The model under review builds one solid part; all positions refer to its coordinate system, in mm. A direction names the side the tool comes from. Give positions to 0.01 mm unless a question says otherwise; leave off trailing zeros. Order: outer loops, then holes, each group sorted by start corner. A loop starts at its lowest first (then second) coordinate and runs counter-clockwise, first axis right, second up. Notation, with made-up numbers: (3.25, 72.25) - (34.25, 72.25) arc R20 ccw to (34.25, 76.25) - close; hole circle Ø7 at (-8.5, 3.5). An arc over 180 degrees is marked (long way). Use CSV: the item, a comma, the result in double quotes.
```python
from build123d import *

# Parameters (mm, degrees)
SKETCH1_R           = 1.5
BOSS_EXTRUDE2_DEPTH = 16
FILLET1_R           = 16
SKETCH2_W           = 30
SKETCH2_H           = 8
CUT_EXTRUDE2_DEPTH  = 93.222557038
SKETCH3_W           = 22.4
SKETCH3_H           = 12.4
CUT_EXTRUDE3_DEPTH  = 93.222557038
SKETCH4_R           = 1.5
CUT_EXTRUDE4_DEPTH  = 88.960218414


with BuildPart() as part:
    # Sketch1 → Boss-Extrude2 (new body)
    with BuildSketch(Plane(origin=(0, 0, 0), x_dir=(1, 0, 0), z_dir=(0, 1, 0))):
        with BuildLine():
            Line((0, -16), (68, -16))
            Line((68, -16), (82.565771817, -7.291481677))
            ThreePointArc((82.565771817, -7.291481677), (84.636633862, -1.128736675), (78.868265673, 1.870233815))
            add(Edge.make_bspline(
                [(78.868265673, 1.870233815), (43.304736125, -17.072492838), (13.642052319, 8.360287586)],
                knots=[0.972219652, 0.972219652, 0.972219652, 1.878474777, 1.878474777, 1.878474777], degree=2))
            ThreePointArc((13.642052319, 8.360287586), (-13.960025096, 7.817780971), (0, -16))
        make_face()
        with Locations(Location((80, -3, 0), (0, 0, 270))):
            Circle(SKETCH1_R, mode=Mode.SUBTRACT)
    extrude(amount=BOSS_EXTRUDE2_DEPTH)

    # Fillet1
    fillet1_edges = [part.edges().sort_by_distance(p)[0] for p in [
        (68, 8, 16),
    ]]
    fillet(fillet1_edges, radius=FILLET1_R)

    # Sketch2 → Cut-Extrude2 (cut, through all)
    with BuildSketch(Plane.XY.offset(16)):
        with Locations((70, 8)):
            Rectangle(SKETCH2_W, SKETCH2_H)
    extrude(amount=-CUT_EXTRUDE2_DEPTH, mode=Mode.SUBTRACT)

    # Sketch3 → Cut-Extrude3 (cut, through all)
    with BuildSketch(Plane.XY.offset(16)):
        with Locations((16.2, 8)):
            Rectangle(SKETCH3_W, SKETCH3_H)
    extrude(amount=-CUT_EXTRUDE3_DEPTH, mode=Mode.SUBTRACT)

    # Sketch4 → Cut-Extrude4 (cut, through all)
    with BuildSketch(Plane.XZ):
        with Locations(Location((0, -10, 0), (0, 0, 270))):
            Circle(SKETCH4_R)
        with Locations(Location((-10, 0, 0), (0, 0, 270))):
            Circle(SKETCH4_R)
        with Locations(Location((0, 10, 0), (0, 0, 270))):
            Circle(SKETCH4_R)
    extrude(amount=-CUT_EXTRUDE4_DEPTH, mode=Mode.SUBTRACT)


solid = part.part
```
Item 1: Take a section at A-A, the plane x = -10. Give the boundary of the cut face in (y, z), and give its area (3 significant figures).
Results list:
outline,"(0, -12.49) - (16, -12.49) - (16, -1.5) - (0, -1.5) - close; (0, 1.5) - (16, 1.5) - (16, 12.49) - (0, 12.49) - close"
area,"352 mm2"
Item 2: Tool access review of faces 5 (the face through (-11.464, 7.888, 0.325)), 6 (the face through (27.4, 8, 9)), 7 (the face through (55, 8, 11)): name each direction out of +Z, -Z, +X, -X, +Y, -Y from which nothing blocks a thin tool from reaching the whole face with its end or side.
Results list:
face 5,"+Y, -Y"
face 6,"+Z, -Z"
face 7,"+Z, -Z, +X"
Item 3: Take a section at B-B, the plane z = -10. Give the boundary of the cut face in (x, y), and give its area (3 significant figures).
Results list:
outline,"(-12.49, 0) - (-1.5, 0) - (-1.5, 16) - (-12.49, 16) - close; (1.5, 0) - (12.49, 0) - (12.49, 1.8) - (5, 1.8) - (5, 14.2) - (12.49, 14.2) - (12.49, 16) - (1.5, 16) - close"
area,"259 mm2"
Item 4: Clearance check with flat-ended pins moving along their axes: pin 1 (4 mm diameter, centred on x = 46, y = 7.5, fed in from -Z); pin 2 (4 mm diameter, centred on x = 27, z = 0, fed in from -Y); pin 3 (4 mm diameter, centred on x = 11, y = 11.5, fed in from -Z); pin 4 (4 mm diameter, centred on y = 2.5, z = -12, fed in from -X). State where each tip first meets the part, or that it passes through.
Results list:
pin 1,"stops at z = 5.89"
pin 2,"stops at y = 0"
pin 3,"passes through"
pin 4,"stops at x = -12.49"
Item 5: Wall thickness on L1, parallel to X at y = 11, z = 0; L2, parallel to Y at x = 13, z = -1; L3, parallel to Y at x = 79, z = -0.5: over which ranges is each line inside the solid? List them lowest first.
Results list:
L1,"x = -16 to -11.5, -8.5 to 5"
L2,"y = 0 to 1.8, 14.2 to 16"
L3,"y = 0 to 4, 12 to 16"
Item 6: Take a section at C-C, the plane z = 10. Give the boundary of the cut face in (x, y), and give its area (3 significant figures).
Results list:
outline,"(-12.49, 0) - (-1.5, 0) - (-1.5, 16) - (-12.49, 16) - close; (1.5, 0) - (78.04, 0) - (78.04, 4) - (55, 4) - (55, 12) - (78.04, 12) - (78.04, 16) - (1.5, 16) - close; hole (5, 1.8) - (27.4, 1.8) - (27.4, 14.2) - (5, 14.2) - close"
area,"938 mm2"
Item 7: Mouldability with a two-part tool opening along X and no side actions: class faces 1 (the face through (0.07, 7.89, 11.5)), 2 (the face through (67.78, 14.03, 15.44)), 3 (the face through (70, 4, 7)), 4 (the face through (14, 14.2, 4)) as pulls with the +X half, pulls with the -X half, needs draft (parallel to the pull), parting line crosses it, or undercut.
Results list:
face 1,"undercut"
face 2,"pulls with the +X half"
face 3,"needs draft"
face 4,"undercut"
Item 8: Take a section at D-D, the plane x = 80. Give the boundary of the cut face in (y, z).
Results list:
outline,"(0, -2) - (4, -2) - (4, 1.5) - (0, 1.5) - close; (0, 4.5) - (4, 4.5) - (4, 8.83) - (0, 8.83) - close; (12, -2) - (16, -2) - (16, 1.5) - (12, 1.5) - close; (12, 4.5) - (16, 4.5) - (16, 8.83) - (12, 8.83) - close"
